Could you check a few things on this drawing? It's one solid part, dimensions in mm from its lowest x, y, z. A direction names the side the tool comes from. Give positions to 0.01 mm unless a question says otherwise; leave off trailing zeros. Order: outer loops, then holes, each group sorted by start corner. A loop starts at its lowest first (then second) coordinate and runs counter-clockwise, first axis right, second up.
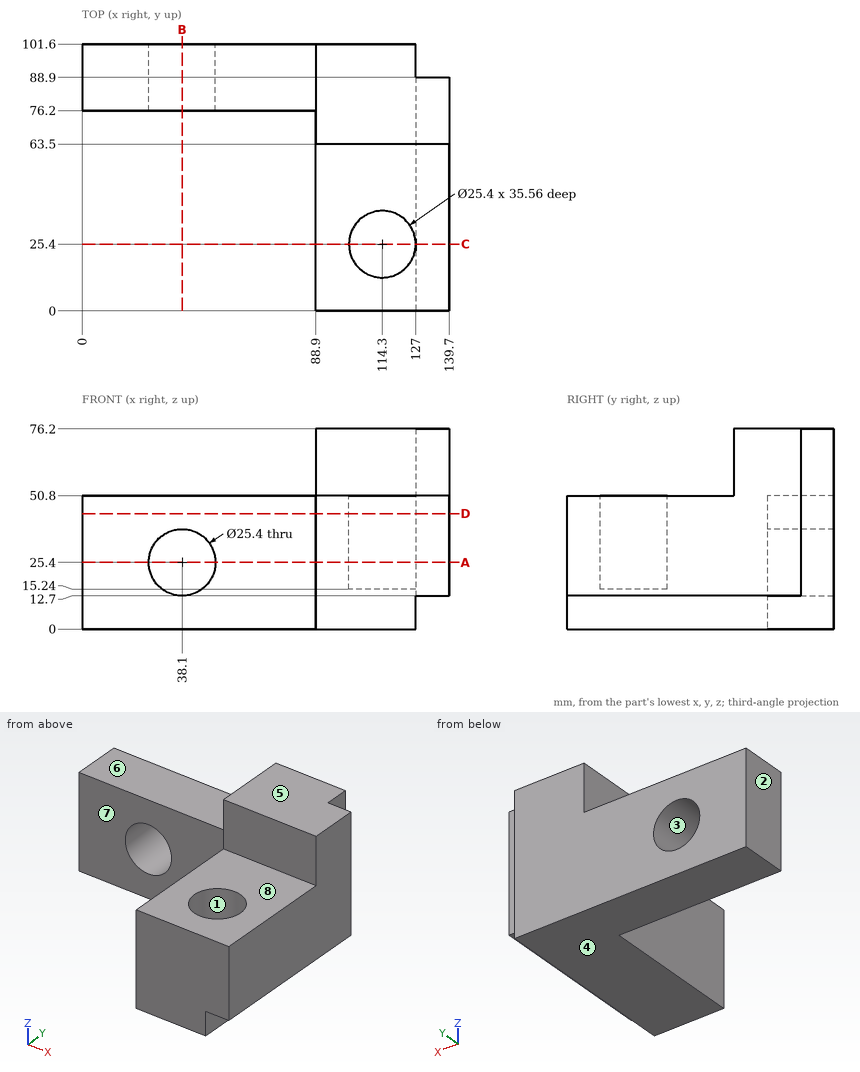
Item 1: For pin 1 (15 mm diameter, centred on x = 38.1, z = 25.4, fed in from -Y); pin 2 (6.5 mm diameter, centred on x = 131.5, z = 30, fed in from +Y); pin 3 (20.5 mm diameter, centred on x = 32.5, y = 91, fed in from +Z); pin 4 (23 mm diameter, centred on y = 52.5, z = 47.5, fed in from -X), each with a flat end and sliding along its axis, tell me the tip position at first contact or that it passes through.
Findings:
pin 1: passes through
pin 2: stops at y = 88.9
pin 3: stops at z = 50.8
pin 4: stops at x = 88.9
Item 2: Imagine slicing it at C-C on y = 25.4. List the corners of the cut face in (x, z) for me, then the cut area to 3 significant figures.
Findings:
outline: (88.9, 0) - (127, 0) - (127, 12.7) - (139.7, 12.7) - (139.7, 50.8) - (127, 50.8) - (127, 15.24) - (101.6, 15.24) - (101.6, 50.8) - (88.9, 50.8) - close
area: 1,520 mm2
Item 3: Imagine slicing it at B-B on x = 38.1. List the corners of the cut face in (y, z) for me.
Findings:
outline: (76.2, 0) - (101.6, 0) - (101.6, 12.7) - (76.2, 12.7) - close; (76.2, 38.1) - (101.6, 38.1) - (101.6, 50.8) - (76.2, 50.8) - close
Item 4: For the marked faces 5, 6, 7 and 8, which set-ups out of +Z, -Z, +X, -X, +Y, -Y let a thin tool reach every point of the face, with its end or its side?
Findings:
face 5: +Z, +X, -X, +Y, -Y
face 6: +Z, -X, +Y, -Y
face 7: +Z, -Z, -X, -Y
face 8: +Z, +X, -X, -Y
Item 5: Please list where these lines run through material, in increasing order: line 1 along X through (y, z) = (91, 25); line 2 along X through (y, z) = (87, 25); line 3 along Y through (x, z) = (114, 37).
Findings:
line 1: x = 0 to 25.41, 50.79 to 127
line 2: x = 0 to 25.41, 50.79 to 139.7
line 3: y = 0 to 12.7, 38.1 to 101.6
Item 6: We'd pull the mould along X, two halves only. Please class the marked faces 1, 2, 3 and 4: +X half, -X half, draft (parallel to the pull), parting line (faces both ways), or undercut.
Findings:
face 1: undercut
face 2: -X half
face 3: undercut
face 4: draft
Item 7: Imagine slicing it at D-D on z = 44. List the corners of the cut face in (x, y) for me.
Findings:
outline: (0, 76.2) - (88.9, 76.2) - (88.9, 0) - (139.7, 0) - (139.7, 88.9) - (127, 88.9) - (127, 101.6) - (0, 101.6) - close; hole circle Ø25.4 at (114.3, 25.4)
Item 8: Imagine slicing it at A-A on z = 25.4. List the corners of the cut face in (x, y) for me.
Findings:
outline: (0, 76.2) - (25.4, 76.2) - (25.4, 101.6) - (0, 101.6) - close; (50.8, 76.2) - (88.9, 76.2) - (88.9, 0) - (139.7, 0) - (139.7, 88.9) - (127, 88.9) - (127, 101.6) - (50.8, 101.6) - close; hole circle Ø25.4 at (114.3, 25.4)
